from build123d import *

# Parameters (mm, degrees)
CROQUIS1_W               = 72
CROQUIS1_H               = 74
SALIENTE_EXTRUIR3_DEPTH  = 4
CROQUIS2_W               = 3
CROQUIS2_H               = 6
SALIENTE_EXTRUIR4_DEPTH  = 7.6
CORTAR_EXTRUIR3_DEPTH    = 83.938591741
CROQUIS5_W               = 5
CROQUIS5_H               = 4
SALIENTE_EXTRUIR5_DEPTH  = 1
CROQUIS9_W               = 72
CROQUIS9_H               = 1.5
SALIENTE_EXTRUIR6_DEPTH  = 8
CROQUIS10_W              = 72
CROQUIS10_H              = 5.9
SALIENTE_EXTRUIR7_DEPTH  = 2
CROQUIS11_W              = 10
CROQUIS11_H              = 4.4
SALIENTE_EXTRUIR10_DEPTH = 7
SALIENTE_EXTRUIR14_DEPTH = 10
CROQUIS15_W              = 18
CROQUIS15_H              = 4.4
SALIENTE_EXTRUIR15_DEPTH = 5
CROQUIS16_W              = 72
CROQUIS16_H              = 40
SALIENTE_EXTRUIR16_DEPTH = 10.5
CROQUIS17_W              = 72
CROQUIS17_H              = 5
SALIENTE_EXTRUIR17_DEPTH = 8
CROQUIS18_W              = 72
CROQUIS18_H              = 8
SALIENTE_EXTRUIR19_DEPTH = 2
CROQUIS19_W              = 72
CROQUIS19_H              = 1
CORTAR_EXTRUIR4_DEPTH    = 14.5
CROQUIS20_W              = 59
CROQUIS20_H              = 7
SALIENTE_EXTRUIR20_DEPTH = 65
CROQUIS26_R              = 1.25
CROQUIS26_R_2            = 1.3
CORTAR_EXTRUIR5_DEPTH    = 10
REDONDEO1_R              = 5
CORTAR_EXTRUIR6_REACH    = 103.4
CROQUIS27_W              = 59
CROQUIS27_H              = 9


with BuildPart() as part:
    # Croquis1 → Saliente-Extruir3 (new body)
    with BuildSketch(Plane.XY):
        with Locations((0, -2.5)):
            Rectangle(CROQUIS1_W, CROQUIS1_H)
    extrude(amount=SALIENTE_EXTRUIR3_DEPTH)

    # Croquis2 → Saliente-Extruir4 (add)
    with BuildSketch(Plane.XY.offset(4)):
        with Locations((-34.5, -36.5)):
            Rectangle(CROQUIS2_W, CROQUIS2_H)
        with Locations((34.5, -36.5)):
            Rectangle(CROQUIS2_W, CROQUIS2_H)
    extrude(amount=SALIENTE_EXTRUIR4_DEPTH)

    # Croquis3 → Cortar-Extruir3 (cut, through all)
    with BuildSketch(Plane.ZY.offset(36)):
        Polygon((4, -39.5), (11.6, -36.5), (11.6, -39.5), align=None)
    extrude(amount=-CORTAR_EXTRUIR3_DEPTH, mode=Mode.SUBTRACT)

    # Croquis5 → Saliente-Extruir5 (add)
    with BuildSketch(Plane.XY.offset(4)):
        with Locations((-33.5, -30.5)):
            Rectangle(CROQUIS5_W, CROQUIS5_H)
        with Locations((33.5, -29.5)):
            Rectangle(CROQUIS5_W, CROQUIS5_H)
    extrude(amount=SALIENTE_EXTRUIR5_DEPTH)

    # Croquis9 → Saliente-Extruir6 (add)
    with BuildSketch(Plane.XY.offset(4)):
        with Locations((0, -26.35)):
            Rectangle(CROQUIS9_W, CROQUIS9_H)
    extrude(amount=SALIENTE_EXTRUIR6_DEPTH)

    # Croquis10 → Saliente-Extruir7 (add)
    with BuildSketch(Plane.XY.offset(12)):
        with Locations((0, -28.55)):
            Rectangle(CROQUIS10_W, CROQUIS10_H)
    extrude(amount=SALIENTE_EXTRUIR7_DEPTH)

    # Croquis11 → Saliente-Extruir10 (add)
    with BuildSketch(Plane.XY.offset(14)):
        with Locations((-31, -29.3)):
            Rectangle(CROQUIS11_W, CROQUIS11_H)
        with Locations((31, -29.3)):
            Rectangle(CROQUIS11_W, CROQUIS11_H)
    extrude(amount=-SALIENTE_EXTRUIR10_DEPTH)

    # Croquis14 → Saliente-Extruir14 (add)
    with BuildSketch(Plane.XY.offset(4)):
        with BuildLine():
            Line((-9, -23.7), (-9, -25.6))
            Line((-9, -25.6), (-2.1, -25.6))
            ThreePointArc((-2.1, -25.6), (-2.656497116, -24.256497116), (-4, -23.7))
            Line((-4, -23.7), (-9, -23.7))
        make_face()
        with BuildLine():
            Line((-9, -21.2), (-9, -22.2))
            Line((-9, -22.2), (-4, -22.2))
            ThreePointArc((-4, -22.2), (-2.22447191, -22.714955647), (-1, -24.1))
            Line((-1, -24.1), (1, -24.1))
            ThreePointArc((1, -24.1), (2.22447191, -22.714955647), (4, -22.2))
            Line((4, -22.2), (9, -22.2))
            Line((9, -22.2), (9, -21.2))
            Line((9, -21.2), (-9, -21.2))
        make_face()
        with BuildLine():
            ThreePointArc((4, -23.7), (2.656497116, -24.256497116), (2.1, -25.6))
            Line((2.1, -25.6), (9, -25.6))
            Line((9, -25.6), (9, -23.7))
            Line((9, -23.7), (4, -23.7))
        make_face()
    extrude(amount=SALIENTE_EXTRUIR14_DEPTH)

    # Croquis15 → Saliente-Extruir15 (add)
    with BuildSketch(Plane.XY.offset(4)):
        with Locations((0, -23.4)):
            Rectangle(CROQUIS15_W, CROQUIS15_H)
    extrude(amount=SALIENTE_EXTRUIR15_DEPTH)

    # Croquis16 → Saliente-Extruir16 (add)
    with BuildSketch(Plane.XY.offset(4)):
        with Locations((0, 14.5)):
            Rectangle(CROQUIS16_W, CROQUIS16_H)
    extrude(amount=SALIENTE_EXTRUIR16_DEPTH)

    # Croquis17 → Saliente-Extruir17 (add)
    with BuildSketch(Plane.XY.offset(14.5)):
        with Locations((0, 32)):
            Rectangle(CROQUIS17_W, CROQUIS17_H)
    extrude(amount=SALIENTE_EXTRUIR17_DEPTH)

    # Croquis18 → Saliente-Extruir19 (add)
    with BuildSketch(Plane(origin=(0, 34.5, 0), x_dir=(1, 0, 0), z_dir=(0, 1, 0))):
        with Locations((0, -18.5)):
            Rectangle(CROQUIS18_W, CROQUIS18_H)
    extrude(amount=SALIENTE_EXTRUIR19_DEPTH)

    # Croquis19 → Cortar-Extruir4 (cut)
    with BuildSketch(Plane(origin=(0, 0, 0), x_dir=(-1, 0, 0), z_dir=(0, 0, -1))):
        with Locations((0, 34)):
            Rectangle(CROQUIS19_W, CROQUIS19_H)
    extrude(amount=-CORTAR_EXTRUIR4_DEPTH, mode=Mode.SUBTRACT)

    # Croquis20 → Saliente-Extruir20 (add)
    with BuildSketch(Plane(origin=(0, 0, 0), x_dir=(-1, 0, 0), z_dir=(0, 0, -1))):
        with Locations((0, -36)):
            Rectangle(CROQUIS20_W, CROQUIS20_H)
    extrude(amount=SALIENTE_EXTRUIR20_DEPTH)

    # Croquis26 → Cortar-Extruir5 (cut)
    with BuildSketch(Plane(origin=(0, -32.5, 0), x_dir=(1, 0, 0), z_dir=(0, 1, 0))):
        with Locations(Location((-18, 5, 0), (0, 0, 270))):
            Circle(CROQUIS26_R)
        with Locations(Location((18, 5, 0), (0, 0, 270))):
            Circle(CROQUIS26_R)
        Polygon((20.192818919, 53.25), (-22, 53.25), (-22, 33.25), (-12, 33.25), (-12, 7.5), (28, 7.5), (28, 32.5), (20.192818919, 32.5), align=None)
        with Locations(Location((23, 5, 0), (0, 0, 270))):
            Circle(CROQUIS26_R_2)
        with Locations(Location((-23, 5, 0), (0, 0, 270))):
            Circle(CROQUIS26_R_2)
        with Locations(Location((-24.5, 43.25, 0), (0, 0, 270))):
            Circle(CROQUIS26_R)
    extrude(amount=-CORTAR_EXTRUIR5_DEPTH, mode=Mode.SUBTRACT)

    # Redondeo1
    redondeo1_edges = [part.edges().sort_by_distance(p)[0] for p in [
        (20.192818919, -36, -32.5),
        (-12, -36, -33.25),
    ]]
    fillet(redondeo1_edges, radius=REDONDEO1_R)

    # Croquis27 → Cortar-Extruir6 (cut, up to next)
    with BuildSketch(Plane(origin=(0, -32.5, 0), x_dir=(1, 0, 0), z_dir=(0, 1, 0)), mode=Mode.PRIVATE) as cortar_extruir6_sk1:
        with Locations((0, 60.5)):
            Rectangle(CROQUIS27_W, CROQUIS27_H)
    cortar_extruir6_tool1 = extrude(cortar_extruir6_sk1.sketch, amount=-CORTAR_EXTRUIR6_REACH, mode=Mode.PRIVATE) & part.part
    add(cortar_extruir6_tool1.solids().sort_by_distance((0, -32.5, -60.5))[0], mode=Mode.SUBTRACT)


solid = part.part
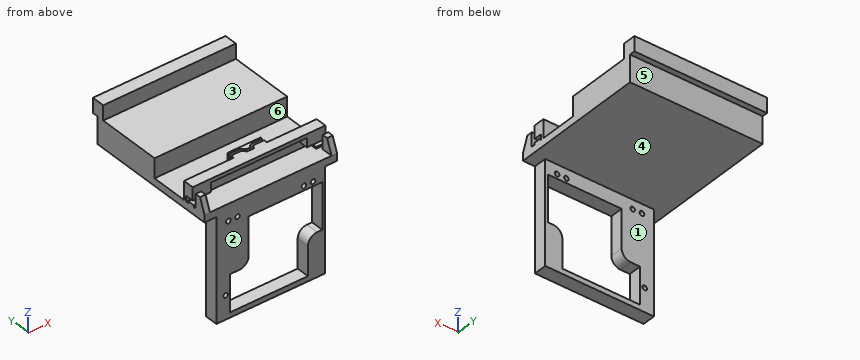
Source: CAD feature listing. Evaluate the final solid. Frame: model axes, mm. Face numbers are marked on the shaded views. A direction names the side the tool comes from. Round coordinates to 2 decimals unless told otherwise and drop trailing zeros. Write each loop counter-clockwise with the first axis right and the second up, starting at its lowest first coordinate (ties: lowest second). Pieces come first, ordered by that corner, then holes. Notation, with made-up numbers: M -28.75,-23.75 L -12.75,-23.75 A25 ccw -12.75,9.25 Z; hole C 60.5,16 d4. An arc over 180 degrees is marked long. One line per item, written item: value. Start each with the question number.
Item 1: Section query C-C (x = -10.5). Return the cut outline in (y, z).
Item 2: Section query B-B (x = 18). Return the cut outline in (y, z).
Item 3: Pin query (flat end, axial travel): pin 1 (2 mm diameter, centred on x = -2.5, y = -35, fed in from +Z); pin 2 (0.8 mm diameter, centred on x = -33.5, z = 4.5, fed in from +Y); pin 3 (5 mm diameter, centred on x = -28.5, z = -35.5, fed in from +Y); pin 4 (2 mm diameter, centred on x = -18, z = -5, fed in from +Y). Return the tip coordinate at first contact, or that it passes through.
Item 4: Section query D-D (z = -23). Return the cut outline in (x, y), plus the area to 3 significant figures.
Item 5: Set-up query: the marked faces 1, 2 and 3. Return all of +Z, -Z, +X, -X, +Y, -Y with unobstructed straight access to the full face (end or side cutting, diameter ignored); none if empty.
Item 6: Section query A-A (z = -43.25). Return the cut outline in (x, y).
Item 7: Mould query, pull axis Y, two halves, no side actions, for the marked faces 4, 5 and 6. Classes: pulls with the +Y half, pulls with the -Y half, needs draft (parallel to the pull), parting line crosses it, or undercut.
Item 8: Ray query, L1, parallel to X at y = -36.5, z = -5; L2, parallel to Z at x = -20, y = -28.5; L3, parallel to X at y = -33, z = -14.5. Return the intervals inside material, ascending. Write a range as from..to.
Result set:
1. outline: M -39.5,-56 L -32.5,-56 L -32.5,-53.25 L -39.5,-53.25 Z; M -39.5,-7.5 L -32.5,-7.5 L -32.5,0 L 33.5,0 L 33.5,14.5 L 36.5,14.5 L 36.5,22.5 L 29.5,22.5 L 29.5,14.5 L -5.5,14.5 L -5.5,4 L -25.6,4 L -25.6,14 L -31.5,14 L -31.5,12 L -27.1,12 L -27.1,4 L -39.5,4 Z
2. outline: M -39.5,-56 L -32.5,-56 L -32.5,-53.25 L -39.5,-53.25 Z; M -39.5,-7.5 L -32.5,-7.5 L -32.5,-6.25 L -39.5,-6.25 Z; M -39.5,-3.75 L -32.5,-3.75 L -32.5,0 L 33.5,0 L 33.5,14.5 L 36.5,14.5 L 36.5,22.5 L 29.5,22.5 L 29.5,14.5 L -5.5,14.5 L -5.5,4 L -25.6,4 L -25.6,14 L -31.5,14 L -31.5,12 L -27.1,12 L -27.1,4 L -39.5,4 Z
3. pin 1: stops at z = 4
3. pin 2: stops at y = 33.5
3. pin 3: stops at y = -32.5
3. pin 4: passes through
4. outline: M -29.5,-39.5 L -12,-39.5 L -12,-32.5 L -29.5,-32.5 Z; M 28,-39.5 L 29.5,-39.5 L 29.5,-32.5 L 28,-32.5 Z
4. area: 133 mm²
5. face 1: -Z, +X, -X, +Y
5. face 2: +Z, -Z, +X, -X, -Y
5. face 3: +Z, +X, -X, -Y
6. outline: M -29.5,-39.5 L -25.75,-39.5 L -25.75,-32.5 L -29.5,-32.5 Z; M -23.25,-39.5 L -22,-39.5 L -22,-32.5 L -23.25,-32.5 Z; M 20.19,-39.5 L 29.5,-39.5 L 29.5,-32.5 L 20.19,-32.5 Z
7. face 4: needs draft
7. face 5: pulls with the +Y half
7. face 6: undercut
8. L1: x = -29.5..-24.3, -21.7..-19.25, -16.75..16.75, 19.25..21.7, 24.3..29.5
8. L2: z = 0..4, 12..14
8. L3: x = -29.5..-12, 28..29.5
